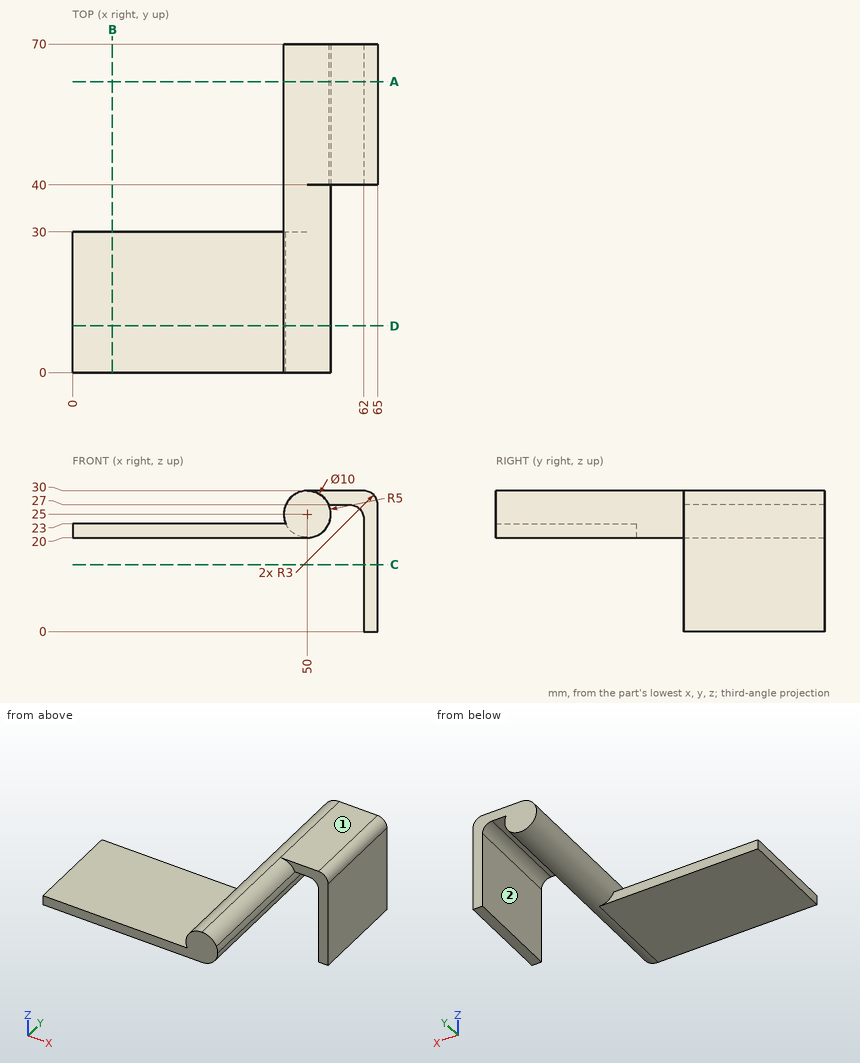
Verification items for this drawing (mm, ordinates from the low corner). A direction names the side the tool comes from. Round coordinates to 2 decimals unless told otherwise and drop trailing zeros. Order: outer loops, then holes, each group sorted by start corner. A loop starts at its lowest first (then second) coordinate and runs counter-clockwise, first axis right, second up. Notation, with made-up numbers: (29, 55) - (82, 55) arc R31 ccw to (82, 93) - close; hole circle Ø11 at (-21, 76.5). An arc over 180 degrees is marked (long way). Use CSV: the item, a comma, the result in double quotes.
(1) Thickness scan on probe 1 along X at (y, z) = (40.5, 3); probe 2 along X at (y, z) = (38, 24.75); probe 3 along Z at (x, y) = (31.5, 13.5). Record the ranges inside material, lowest first. Write a range as from..to.
Entries:
probe 1,"62..65"
probe 2,"45.01..54.99"
probe 3,"20..23"
(2) Section check A-A on y = 62. Record the boundary of the cut face in (x, z).
Entries:
outline,"(50, 30) arc R5 ccw (long way) to (55, 25) arc R5 ccw to (54.58, 27) - (59, 27) arc R3 cw to (62, 24) - (62, 0) - (65, 0) - (65, 27) arc R3 ccw to (62, 30) - close"
(3) Section check D-D on y = 10. Record the boundary of the cut face in (x, z).
Entries:
outline,"(0, 20) - (50, 20) arc R5 ccw to (55, 25) arc R5 ccw to (54.58, 27) arc R5 ccw to (45.42, 23) - (0, 23) - close"
(4) Access from +Z, -Z, +X, -X, +Y, -Y to the whole of each face (thin tool, end or side, straight path). Record for the marked faces 1 and 2.
Entries:
face 1,"+Z, +X, -X, +Y, -Y"
face 2,"-Z, +Y, -Y"
(5) Section check B-B on x = 8.5. Record the boundary of the cut face in (y, z).
Entries:
outline,"(0, 20) - (30, 20) - (30, 23) - (0, 23) - close"
(6) Gauge pin test, flat ends, axial feed: pin 1 Ø5 at (x, y) = (56, 52.5) entering from -Z; pin 2 Ø1 at (x, y) = (21.5, 24.5) entering from +Z; pin 3 Ø7.5 at (x, z) = (58, 11.5) entering from -Y; pin 4 Ø24 at (x, y) = (16, 9) entering from -Z. Record the tip position at first contact, or that the pin passes through.
Entries:
pin 1,"z = 21.43"
pin 2,"z = 23"
pin 3,"through"
pin 4,"z = 20"
(7) Section check C-C on z = 14.25. Record the boundary of the cut face in (x, y), and give its area (3 significant figures).
Entries:
outline,"(62, 40) - (65, 40) - (65, 70) - (62, 70) - close"
area,"90.0 mm^2"
